Autodesk Inventor part; units mm, degrees
ref_plane "YZ Plane" through (0, 0, 0) normal (1, 0, 0) x (0, 1, 0)
ref_plane "XZ Plane" through (0, 0, 0) normal (0, 1, 0) x (-1, 0, 0)
ref_plane "XY Plane" through (0, 0, 0) normal (0, 0, 1) x (1, 0, 0)
sketch "Sketch1" plane through (0, 0, 0) normal (0, 1, 0) x (-1, 0, 0)
  line L0 (0, -3.175) -> (0, -155.575)
  line L1 (-3.175, -158.75) -> (-63.5, -158.75)
  line L2 (-3.175, 0) -> (-63.5, 0)
  line L3 (-63.5, -161.925) -> (0, -161.925)
  line L4 (3.175, -158.75) -> (3.175, 0)
  line L5 (0, 3.175) -> (-63.5, 3.175)
  line L6 (-63.5, 0) -> (-63.5, 3.175)
  line L7 (-63.5, -161.925) -> (-63.5, -158.75)
  arc A0 (3.175, 0) -> (0, 3.175) centre (0, 0) ccw
  arc A1 (0, -3.175) -> (-3.175, 0) centre (-3.175, -3.175) ccw
  arc A2 (-3.175, -158.75) -> (0, -155.575) centre (-3.175, -155.575) ccw
  arc A3 (0, -161.925) -> (3.175, -158.75) centre (0, -158.75) ccw
  point P0 (0, 0)
  point P1 (0, -158.75)
  dimension "d0" = 158.75
  dimension "d1" = 63.5
  dimension "d2" = 63.5
  dimension "d3" = 3.175
  dimension "d4" = 3.175
extrude "Extrusion1" add sketch "Sketch1" along normal blind 76.2
sketch "Sketch2" plane through (0, 0, 3.175) normal (0, 0, 1) x (1, 0, 0)
  circle A0 centre (31.75, 12.7) radius 6.35
  line L0 (63.5, 0) -> (63.5, 76.2)
  line L1 (0, 76.2) -> (63.5, 76.2)
  point P0 (0, 0)
  dimension "d7" = 12.7
  dimension "d8" = 31.75
  dimension "d9" = 63.5
extrude "Extrusion2" cut sketch "Sketch2" against normal through all
properties part number "C chanel Short"
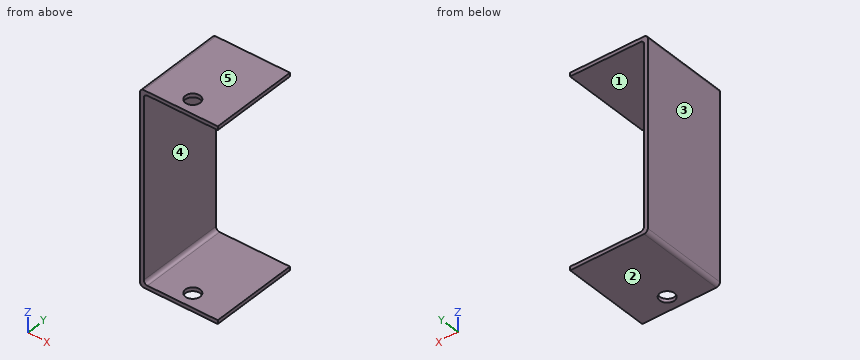
Can you work these out from the model? Positions are in its coordinate system, mm. Face numbers are marked on the shaded views. A direction names the side the tool comes from. Coordinates: 2 decimals unless noted, no trailing zeros. Loops run counter-clockwise (first coordinate to the right, second up) from the corner with the lowest first, then second, coordinate; pieces in that order, holes last. Notation, with made-up numbers: (21, -19) - (68, -19) arc R30 cw to (68, 17) - close; hole circle Ø3 at (-26, 63.25). An arc over 180 degrees is marked (long way). Put each result on its own line as item: value. Start each with the question number.
Item 1: Suppose I cut it at A-A (x = 31.75). Please give me the cut outline in (y, z) (3 decimals).
Item 2: If we mould it in two halves opening along Z, with no side actions, what happens to the marked faces 3, 4 and 5? For each: +Z half, -Z half, draft (parallel to the pull), parting line (faces both ways), or undercut.
Item 3: Suppose I cut it at B-B (x = 51). Please give me the cut outline in (y, z) (3 decimals).
Item 4: If I drill on line 1 along Z through (x, y) = (11, 62) (3 decimals); line 2 along Y through (x, z) = (31.75, 1.8); line 3 along Z through (x, y) = (3, 5) (3 decimals), over which ranges is the centre line in solid material (lowest first)?
Item 5: Suppose I cut it at D-D (y = 30). Please give me the cut outline in (x, z) (3 decimals).
Item 6: Which directions (+Z, -Z, +X, -X, +Y, -Y) give clear straight access to the entire face, cutting with the end or side of a thin tool? Please do the marked faces 1 and 2.
Item 7: For pin 1 (1 mm diameter, centred on y = 41, z = -144.5, fed in from +X); pin 2 (10 mm diameter, centred on x = 31.75, y = 12.7, fed in from +Z); pin 3 (16.5 mm diameter, centred on x = 31.75, y = 12.7, fed in from +Z) (3 decimals), each with a flat end and sliding along its axis, tell me the tip position at first contact or that it passes through.
Item 8: Suppose I cut it at C-C (y = 12.7). Please give me the cut outline in (x, z) (3 decimals).
Here are the results:
1. outline: (0, -161.925) - (6.35, -161.925) - (6.35, -158.75) - (0, -158.75) - close; (0, 0) - (6.35, 0) - (6.35, 3.175) - (0, 3.175) - close; (19.05, -161.925) - (76.2, -161.925) - (76.2, -158.75) - (19.05, -158.75) - close; (19.05, 0) - (76.2, 0) - (76.2, 3.175) - (19.05, 3.175) - close
2. face 3: draft
2. face 4: undercut
2. face 5: +Z half
3. outline: (0, -161.925) - (76.2, -161.925) - (76.2, -158.75) - (0, -158.75) - close; (0, 0) - (76.2, 0) - (76.2, 3.175) - (0, 3.175) - close
4. line 1: -161.925 to -158.75, 0 to 3.175
4. line 2: 0 to 6.35, 19.05 to 76.2
4. line 3: -161.925 to -158.745, -0.005 to 3.175
5. outline: (-3.175, -158.75) arc R3.175 ccw to (0, -161.925) - (63.5, -161.925) - (63.5, -158.75) - (3.175, -158.75) arc R3.175 cw to (0, -155.575) - (0, -3.175) arc R3.175 cw to (3.175, 0) - (63.5, 0) - (63.5, 3.175) - (0, 3.175) arc R3.175 ccw to (-3.175, 0) - close
6. face 1: +X, +Y, -Y
6. face 2: -Z, +X, -X, +Y, -Y
7. pin 1: x = 0
7. pin 2: through
7. pin 3: z = 3.175
8. outline: (-3.175, -158.75) arc R3.175 ccw to (0, -161.925) - (25.4, -161.925) - (25.4, -158.75) - (3.175, -158.75) arc R3.175 cw to (0, -155.575) - (0, -3.175) arc R3.175 cw to (3.175, 0) - (25.4, 0) - (25.4, 3.175) - (0, 3.175) arc R3.175 ccw to (-3.175, 0) - close; (38.1, -161.925) - (63.5, -161.925) - (63.5, -158.75) - (38.1, -158.75) - close; (38.1, 0) - (63.5, 0) - (63.5, 3.175) - (38.1, 3.175) - close
